Design review of the part built by this model. Coordinates are the model's own, in mm. Face numbers are marked on the shaded views. A direction names the side the tool comes from. Coordinates: 2 decimals unless noted, no trailing zeros. Order: outer loops, then holes, each group sorted by start corner. A loop starts at its lowest first (then second) coordinate and runs counter-clockwise, first axis right, second up. Notation, with made-up numbers: (-27.75, -39.75) -> (29.25, -39.75) arc R19 ccw to (29.25, -20.75) -> close; hole circle Ø6 at (82.5, 2). An arc over 180 degrees is marked (long way). Use a Markdown table: item, result. Add a question column.
Q1. Add section B-B (y = -35). State the section outline as (x, z) points.
Q2. Add section A-A (z = 0). State the section outline as (x, y) points.
Q3. Insertion check: pin 1 (2 mm diameter, centred on x = 10, z = -2, fed in from +Y). The pin has a flat end and moves straight along its axis. Give the tip position at first contact, or say it passes through.
Q4. Add section D-D (y = 36.5). State the section outline as (x, z) points.
Q5. Machinability: for the marked faces 1 and 2, which of the approach directions +Z, -Z, +X, -X, +Y, -Y give a long, thin tool a straight path to every point of the face, cutting with its end or side? Answer none if there is none.
Q6. Add section C-C (z = -4). State the section outline as (x, y) points (3 decimals).
Q7. Wall thickness on probe 1 along Z at (x, y) = (3.3, -30) (3 decimals); probe 2 along X at (y, z) = (-35, -4.15); probe 3 along X at (y, z) = (-38.9, 0): over which ranges is each line inside the solid? List them lowest first.
from build123d import *

# Parameters (mm, degrees)
SKETCH_1_W                      = 14
SKETCH_1_H                      = 80
EXTRUDE_1_DEPTH                 = 5
SKETCH_14_W                     = 14
SKETCH_14_H                     = 10
EXTRUDE_2_DEPTH                 = 7
HOLE_WIZARD_M2_5_1_D            = 2.9
HOLE_WIZARD_M2_5_1_CSINK_D      = 5.5
HOLE_WIZARD_M2_5_1_CSINK_ANGLE  = 90
SKETCH_9_W                      = 1.025
SKETCH_9_H                      = 5
HOLE_WIZARD_M2_5_1_2_AT_2_COUNT = 2
HOLE_WIZARD_M2_5_1_2_AT_2_PITCH = 8
SKETCH_15_R                     = 2
CUT_EXTRUDE_2_DEPTH             = 43.343830719
F_1_0MM_2_REACH                 = 46.045
F_1_0MM_2_BORE_R                = 1.35
F_1_0MM_1_REACH                 = 83.197
F_1_0MM_1_BORE_R                = 1.35


with BuildPart() as part:
    # 草圖1 → 填料-伸長1 (new body)
    with BuildSketch(Plane(origin=(0, 0, 0), x_dir=(0, 0, -1), z_dir=(1, 0, 0))):
        Rectangle(SKETCH_1_W, SKETCH_1_H)
    extrude(amount=EXTRUDE_1_DEPTH)

    # 草圖14 → 填料-伸長2 (add)
    with BuildSketch(Plane(origin=(5, 0, 0), x_dir=(0, 0, -1), z_dir=(1, 0, 0))):
        with Locations((0, -35)):
            Rectangle(SKETCH_14_W, SKETCH_14_H)
    extrude(amount=EXTRUDE_2_DEPTH)

    # Hole Wizard M2.5 _1 (through all)
    with Locations(Plane(origin=(5, 0, 0), x_dir=(0, 0, -1), z_dir=(1, 0, 0))):
        with Locations((0, 36.5), (0, 28.5)):
            CounterSinkHole(HOLE_WIZARD_M2_5_1_D / 2, HOLE_WIZARD_M2_5_1_CSINK_D / 2, counter_sink_angle=HOLE_WIZARD_M2_5_1_CSINK_ANGLE)

    # 草圖9 → Hole Wizard M2.5 _1 2 (revolve, cut)
    with BuildSketch(Plane(origin=(5, -30, -4), x_dir=(0, 0, -1), z_dir=(0, 1, 0))):
        with Locations((0.5125, 2.5)):
            Rectangle(SKETCH_9_W, SKETCH_9_H)
    hole_wizard_m2_5_1_2 = revolve(axis=Axis((11.35, -30, -4), (-1, 0, 0)), mode=Mode.SUBTRACT)

    # Hole Wizard M2.5 _1 2 at 2: Hole Wizard M2.5 _1 2 ×2
    with Locations(*[(0, 0, i * HOLE_WIZARD_M2_5_1_2_AT_2_PITCH) for i in range(1, HOLE_WIZARD_M2_5_1_2_AT_2_COUNT)]):
        add(hole_wizard_m2_5_1_2, mode=Mode.SUBTRACT)

    # 草圖15 → 除料-伸長2 (cut, through all)
    with BuildSketch(Plane.ZY):
        with Locations((0, -35)):
            Circle(SKETCH_15_R)
    extrude(amount=-CUT_EXTRUDE_2_DEPTH, mode=Mode.SUBTRACT)

    # Ø1.0mm 定位孔2 bore → Ø1.0mm 定位孔2 (cut, up to next)
    with BuildSketch(Plane(origin=(0, 0, -7), x_dir=(-1, 0, 0), z_dir=(0, 0, -1)), mode=Mode.PRIVATE) as f_1_0mm_2_sk1:
        with Locations((-5, -35)):
            Circle(F_1_0MM_2_BORE_R)
    f_1_0mm_2_tool1 = extrude(f_1_0mm_2_sk1.sketch, amount=-F_1_0MM_2_REACH, mode=Mode.PRIVATE) & part.part
    f_1_0mm_2 = f_1_0mm_2_tool1.solids().sort_by_distance((5, -35, -7))[0]
    add(f_1_0mm_2, mode=Mode.SUBTRACT)

    # 鏡射2: Ø1.0mm 定位孔2 across plane
    add(f_1_0mm_2.mirror(Plane.XY), mode=Mode.SUBTRACT)

    # Ø1.0mm 定位孔1 bore → Ø1.0mm 定位孔1 (cut, up to next)
    with BuildSketch(Plane(origin=(0, -40, 0), x_dir=(-1, 0, 0), z_dir=(0, -1, 0)), mode=Mode.PRIVATE) as f_1_0mm_1_sk1:
        with Locations((-8, 0)):
            Circle(F_1_0MM_1_BORE_R)
    f_1_0mm_1_tool1 = extrude(f_1_0mm_1_sk1.sketch, amount=-F_1_0MM_1_REACH, mode=Mode.PRIVATE) & part.part
    add(f_1_0mm_1_tool1.solids().sort_by_distance((8, -40, 0))[0], mode=Mode.SUBTRACT)


solid = part.part
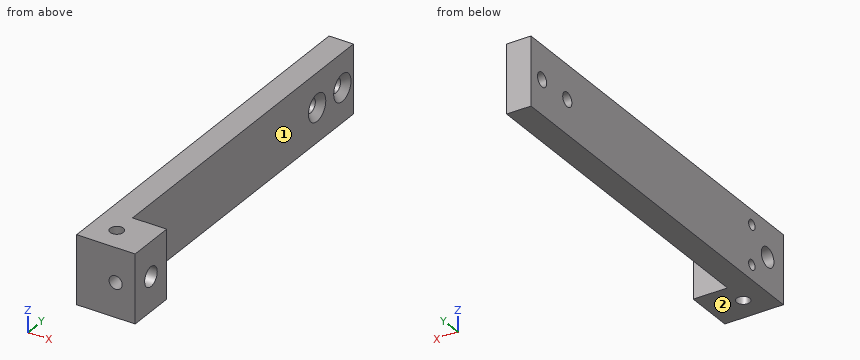
Established:
| question | item | result |
|---|---|---|
| 1 | outline | (0, -7) -> (3.65, -7) -> (3.65, -2) -> (0, -2) -> close; (0, 2) -> (3.65, 2) -> (3.65, 7) -> (0, 7) -> close; (6.35, -7) -> (12, -7) -> (12, -2) -> (6.35, -2) -> close; (6.35, 2) -> (12, 2) -> (12, 7) -> (6.35, 7) -> close |
| 2 | outline | (0, -40) -> (6.65, -40) -> (6.65, -37) -> (0, -37) -> close; (0, -33) -> (12, -33) -> (12, -30) -> (5, -30) -> (5, 25.75) -> (3.7, 27.05) -> (0, 27.05) -> close; (0, 29.95) -> (3.7, 29.95) -> (5, 31.25) -> (5, 33.75) -> (3.7, 35.05) -> (0, 35.05) -> close; (0, 37.95) -> (3.7, 37.95) -> (5, 39.25) -> (5, 40) -> (0, 40) -> close; (9.35, -40) -> (12, -40) -> (12, -37) -> (9.35, -37) -> close |
| 3 | pin 1 | y = -30 |
| 4 | outline | (0, -7) -> (5, -7) -> (5, -2.75) -> (3.7, -1.45) -> (0, -1.45) -> close; (0, 1.45) -> (3.7, 1.45) -> (5, 2.75) -> (5, 7) -> (0, 7) -> close |
| 5 | face 1 | +Z, -Z, +X, +Y |
| 5 | face 2 | -Z, +X, -X, +Y, -Y |
| 6 | outline | (0, -40) -> (12, -40) -> (12, -30) -> (5, -30) -> (5, -31.025) -> (0, -31.025) -> close; (0, -28.975) -> (5, -28.975) -> (5, 40) -> (0, 40) -> close; hole circle Ø2.7 at (5, -35) |
| 7 | probe 1 | -7 to -5.025, -2.975 to 2.975, 5.025 to 7 |
| 7 | probe 2 | 0 to 3.65, 6.35 to 12 |
| 7 | probe 3 | 0 to 6.65, 9.35 to 12 |
